Can you work these out from the model? Positions are in its coordinate system, mm. Face numbers are marked on the shaded views. A direction names the side the tool comes from. Coordinates: 2 decimals unless noted, no trailing zeros. Loops run counter-clockwise (first coordinate to the right, second up) from the corner with the lowest first, then second, coordinate; pieces in that order, holes last. Notation, with made-up numbers: M 76,82.25 L 133,82.25 A23 ccw 133,104.25 Z; hole C 85.5,10.5 d7. An arc over 180 degrees is marked long. Answer as a JSON object with one key per item and string values. Group by question number.
Item 1: Suppose I cut it at A-A (z = 25). Write out the boundary of the cut face in (x, y).
Item 2: Suppose I cut it at D-D (y = -38). Write out the boundary of the cut face in (x, z).
Item 3: If I drill on line 1 (Y direction, x = -11, z = 3.5); line 2 (X direction, y = 0, z = 23); line 3 (Y direction, x = -11, z = 5), over which ranges is the centre line in solid material (lowest first)?
Item 4: Which directions (+Z, -Z, +X, -X, +Y, -Y) give clear straight access to the entire face, cutting with the end or side of a thin tool? Please do the marked faces 1, 2 and 3.
Item 5: Suppose I cut it at C-C (z = 3). Write out the boundary of the cut face in (x, y).
Item 6: We'd pull the mould along X, two halves only. Please class the marked faces 4, 5 and 6: +X half, -X half, draft (parallel to the pull), parting line (faces both ways), or undercut.
Item 7: I'm going to push flat-ended pins straight in: pin 1 Ø5.5 at (x, y) = (1, 33.5) entering from +Z; pin 2 Ø15 at (x, z) = (10, 19.5) entering from -Y; pin 3 Ø5 at (x, y) = (8, -10.5) entering from -Z; pin 4 Ø12 at (y, z) = (9, 31) entering from +X. Where does each tip first touch, or does it pass through?
Item 8: Suppose I cut it at B-B (y = 0). Write out the boundary of the cut face in (x, z), then the cut area to 3 significant figures.
```python
from build123d import *

# Parameters (mm, degrees)
F0_W     = 11
F0_H     = 30
F1_DEPTH = 24
F3_DEPTH = 11
F4_R     = 2.5
F4_R_2   = 5
F5_DEPTH = 41.001
F6_R     = 13
F7_R     = 5
F8_R     = 2


with BuildPart() as f1:
    # F0 (on Right) → F1 (new body, symmetric)
    with BuildSketch(Plane.YZ):
        with Locations((45.5, 26)):
            Rectangle(F0_W, F0_H)
        with BuildLine():
            ThreePointArc((27.9105714739, 11), (29.4730143031, 5.5983415304), (30, 0))
            Line((30, 0), (51, 0))
            Line((51, 0), (51, 11))
            Line((51, 11), (40, 11))
            Line((40, 11), (27.9105714739, 11))
        make_face()
        with BuildLine():
            ThreePointArc((-15.4919333848, 11), (0, 19), (15.4919333848, 11))
            Line((15.4919333848, 11), (27.9105714739, 11))
            ThreePointArc((27.9105714739, 11), (0, 30), (-27.9105714739, 11))
            Line((-27.9105714739, 11), (-15.4919333848, 11))
        make_face()
        with BuildLine():
            ThreePointArc((15.4919333848, 11), (18.1017503893, 5.7729223833), (19, 0))
            Line((19, 0), (30, 0))
            ThreePointArc((30, 0), (29.4730143031, 5.5983415304), (27.9105714739, 11))
            Line((27.9105714739, 11), (15.4919333848, 11))
        make_face()
        with BuildLine():
            Line((-30, 0), (-19, 0))
            ThreePointArc((-19, 0), (-18.1017503893, 5.7729223833), (-15.4919333848, 11))
            Line((-15.4919333848, 11), (-27.9105714739, 11))
            ThreePointArc((-27.9105714739, 11), (-29.4730143031, 5.5983415304), (-30, 0))
        make_face()
        with BuildLine():
            Line((-56, 0), (-30, 0))
            ThreePointArc((-30, 0), (-29.4730143031, 5.5983415304), (-27.9105714739, 11))
            Line((-27.9105714739, 11), (-56, 11))
            Line((-56, 11), (-56, 0))
        make_face()
    extrude(amount=F1_DEPTH, both=True)

    # F2 (on face) → F3 (cut, through all)
    with BuildSketch(Plane(origin=(0, 51, 0), x_dir=(-1, 0, 0), z_dir=(0, 1, 0))):
        with BuildLine():
            ThreePointArc((-6.5, 23), (-4.5961940777, 27.5961940777), (0, 29.5))
            Line((0, 29.5), (0, 41))
            Line((0, 41), (-6.5, 41))
            Line((-6.5, 41), (-6.5, 23))
        make_face()
        with BuildLine():
            ThreePointArc((-6.5, 23), (-4.5961940777, 18.4038059223), (0, 16.5))
            Line((0, 16.5), (0, 29.5))
            ThreePointArc((0, 29.5), (-4.5961940777, 27.5961940777), (-6.5, 23))
        make_face()
        with BuildLine():
            Line((0, 29.5), (0, 16.5))
            ThreePointArc((0, 16.5), (4.5961940777, 18.4038059223), (6.5, 23))
            ThreePointArc((6.5, 23), (4.5961940777, 27.5961940777), (0, 29.5))
        make_face()
        with BuildLine():
            Line((0, 41), (0, 29.5))
            ThreePointArc((0, 29.5), (4.5961940777, 27.5961940777), (6.5, 23))
            Line((6.5, 23), (6.5, 41))
            Line((6.5, 41), (0, 41))
        make_face()
    extrude(amount=-F3_DEPTH, mode=Mode.SUBTRACT)

    # F4 (on Top) → F5 (cut, through all)
    with BuildSketch(Plane.XY):
        Circle(F4_R)
        with Locations((11, -41.955285737)):
            Circle(F4_R_2)
        with Locations((-11, -41.955285737)):
            Circle(F4_R_2)
    extrude(amount=F5_DEPTH, mode=Mode.SUBTRACT)

    # F6
    f6_edges = [f1.edges().sort_by_distance(p)[0] for p in [
        (-24, -56, 5.5),
        (24, -56, 5.5),
    ]]
    fillet(f6_edges, radius=F6_R)

    # F7
    f7_edges = [f1.edges().sort_by_distance(p)[0] for p in [
        (-24, 45.5, 41),
        (24, 45.5, 41),
    ]]
    fillet(f7_edges, radius=F7_R)

    # F8
    f8_edges = [f1.edges().sort_by_distance(p)[0] for p in [
        (0, -27.910571, 11),
        (0, 27.910571, 11),
    ]]
    fillet(f8_edges, radius=F8_R)


solid = f1.part
```
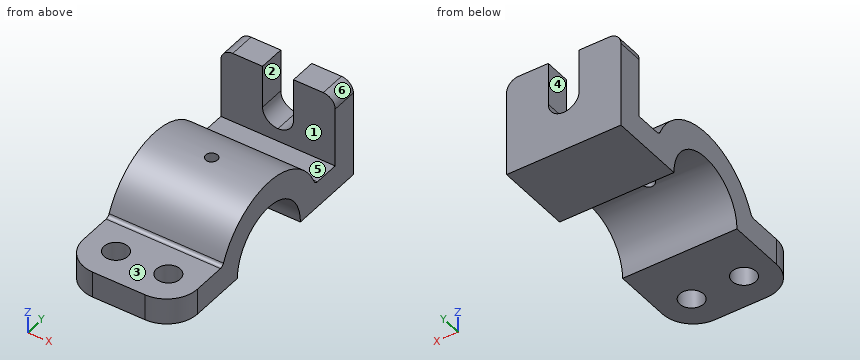
From the geometry:
{
 "1": {"outline": "M -24,-16.58 L 24,-16.58 L 24,16.58 L -24,16.58 Z; M -24,40 L -6.5,40 L -6.5,51 L -24,51 Z; M 6.5,40 L 24,40 L 24,51 L 6.5,51 Z; hole C 0,0 d5"},
 "2": {"outline": "M -24,0 L -14.06,0 L -14.06,11 L -24,11 Z; M -7.94,0 L 7.94,0 L 7.94,11 L -7.94,11 Z; M 14.06,0 L 24,0 L 24,11 L 14.06,11 Z"},
 "3": {"line 1": "-56 to -46.96, -36.96 to -18.67, 18.67 to 51", "line 2": "-24 to -2.5, 2.5 to 24", "line 3": "-56 to -46.96, -36.96 to -18.33, 18.33 to 51"},
 "4": {"face 1": "+Z, +X, -X", "face 2": "+Z, +Y", "face 3": "+Z, +X, -X, -Y"},
 "5": {"outline": "M -24,-43 A13 ccw -11,-56 L 11,-56 A13 ccw 24,-43 L 24,-18.76 L -24,-18.76 Z; M -24,18.76 L 24,18.76 L 24,51 L -24,51 Z; hole C -11,-41.96 d10; hole C 11,-41.96 d10"},
 "6": {"face 4": "undercut", "face 5": "draft", "face 6": "+X half"},
 "7": {"pin 1": "z = 11", "pin 2": "y = -27.51", "pin 3": "z = 13.86", "pin 4": "x = 24"},
 "8": {"outline": "M -24,19 L -2.5,19 L -2.5,30 L -24,30 Z; M 2.5,19 L 24,19 L 24,30 L 2.5,30 Z", "area": "473 mm2"}
}
